Geometry: final body of the model. Coordinates: model frame, mm. Give positions to 0.01 mm unless a question says otherwise; leave off trailing zeros. Loops run counter-clockwise (first coordinate to the right, second up) from the corner with the lowest first, then second, coordinate; pieces in that order, holes last. Notation, with made-up numbers: (-7, 71.25) -> (21, 71.25) arc R33 cw to (21, 102.25) -> close; hole circle Ø2 at (49.5, 39.5). An arc over 180 degrees is marked (long way). Answer in a Markdown table with one row per item. Add a question column.
from build123d import *

# Parameters (mm, degrees)
BOSS_EXTRUDE1_DEPTH = 6.35
SKETCH3_R           = 3.175
CUT_EXTRUDE1_DEPTH  = 27.940768363


with BuildPart() as part:
    # Sketch2 → Boss-Extrude1 (new body)
    with BuildSketch(Plane.XY):
        with BuildLine():
            Line((19.05, -6.35), (-19.05, -6.35))
            ThreePointArc((-19.05, -6.35), (-25.4, 0), (-19.05, 6.35))
            Line((-19.05, 6.35), (19.05, 6.35))
            ThreePointArc((19.05, 6.35), (25.4, 0), (19.05, -6.35))
        make_face()
    extrude(amount=BOSS_EXTRUDE1_DEPTH)

    # Sketch3 → Cut-Extrude1 (cut, through all)
    with BuildSketch(Plane.XY.offset(6.35)):
        with Locations((-19.05, 0)):
            Circle(SKETCH3_R)
        Circle(SKETCH3_R)
        with Locations((19.05, 0)):
            Circle(SKETCH3_R)
    extrude(amount=-CUT_EXTRUDE1_DEPTH, mode=Mode.SUBTRACT)


solid = part.part
(1) Cut plane B-B on x = 0. Return the cut outline in (y, z) (3 decimals).
(2) Cut plane D-D on x = 20.5. Return the cut outline in (y, z).
(3) Material intervals for line 1 along X through (y, z) = (0.25, 1.25); line 2 along Y through (x, z) = (0, 1.5) (3 decimals), sorted ascending. Write a range as from..to.
(4) Cut plane C-C on z = 3.5. Return the cut outline in (x, y) (3 decimals).
(5) Pin query (flat end, axial travel): pin 1 Ø4 at (x, y) = (19.05, 0) entering from -Z (1 decimal); pin 2 Ø4 at (x, y) = (19, 1.5) entering from -Z; pin 3 Ø2 at (y, z) = (1.5, 4.5) entering from +X. Return the tip coordinate at first contact, or that it passes through.
(6) Draft query along X for faces 1 (the cylindrical face through (-16.02, 0.95, 3.22)), 2 (the cylindrical face through (-0.69, -3.1, 3.22)), 3 (the flat face through (0, 4, 0)), 4 (the cylindrical face through (25.4, 0.1, 3.1)). Return one class per face: +X half, -X half, draft (parallel to the pull), parting line (faces both ways), or undercut.
(7) Cut plane A-A on y = 0. Return the cut outline in (x, z) (3 decimals).
Answer list:
| question | item | result |
|---|---|---|
| 1 | outline | (-6.35, 0) -> (-3.175, 0) -> (-3.175, 6.35) -> (-6.35, 6.35) -> close; (3.175, 0) -> (6.35, 0) -> (6.35, 6.35) -> (3.175, 6.35) -> close |
| 2 | outline | (-6.18, 0) -> (-2.82, 0) -> (-2.82, 6.35) -> (-6.18, 6.35) -> close; (2.82, 0) -> (6.18, 0) -> (6.18, 6.35) -> (2.82, 6.35) -> close |
| 3 | line 1 | x = -25.4..-22.22, -15.88..-3.17, 3.17..15.88, 22.22..25.4 |
| 3 | line 2 | y = -6.35..-3.175, 3.175..6.35 |
| 4 | outline | (-19.05, -6.35) -> (19.05, -6.35) arc R6.35 ccw to (19.05, 6.35) -> (-19.05, 6.35) arc R6.35 ccw to start; hole circle Ø6.35 at (-19.05, 0); hole circle Ø6.35 at (0, 0); hole circle Ø6.35 at (19.05, 0) |
| 5 | pin 1 | passes through |
| 5 | pin 2 | stops at z = 0 |
| 5 | pin 3 | stops at x = 25.38 |
| 6 | face 1 | undercut |
| 6 | face 2 | undercut |
| 6 | face 3 | draft |
| 6 | face 4 | +X half |
| 7 | outline | (-25.4, 0) -> (-22.225, 0) -> (-22.225, 6.35) -> (-25.4, 6.35) -> close; (-15.875, 0) -> (-3.175, 0) -> (-3.175, 6.35) -> (-15.875, 6.35) -> close; (3.175, 0) -> (15.875, 0) -> (15.875, 6.35) -> (3.175, 6.35) -> close; (22.225, 0) -> (25.4, 0) -> (25.4, 6.35) -> (22.225, 6.35) -> close |
